Geometry check sheet. Reference: the model listing, model coordinates, mm. Give positions to 0.01 mm unless a question says otherwise; leave off trailing zeros. Write each loop counter-clockwise with the first axis right and the second up, starting at its lowest first coordinate (ties: lowest second). Pieces come first, ordered by that corner, then holes. Notation, with made-up numbers: (-24.5, 15.25) -> (-9.5, 15.25) arc R24 ccw to (-9.5, 30.25) -> close; hole circle Ø9 at (35.25, 30.25). An arc over 180 degrees is marked (long way). Write item = value, one per line. Start each with the question number.
1. Depth check by flat-ended pin: P1, Ø1.5, axis at x = -45.5, z = 27, coming from the +Y side. Enter the tip coordinate at first touch or a pass-through.
2. Thickness scan on line 1 along Z through (x, y) = (-50, -1.1); line 2 along Z through (x, y) = (-51, -0.8); line 3 along X through (y, z) = (-0.9, 45). Record the ranges inside material, lowest first.
3. Cross-section at A-A, the plane y = -0.65. Record the cut outline in (x, z) (3 decimals).
```python
from build123d import *

# Parameters (mm, degrees)
F0_W           = 95.9
F0_H           = 69.7
F1_DEPTH       = 1.54
F2_R           = 7
F3_D           = 2.8448
F3_CSINK_D     = 6.35
F3_CSINK_ANGLE = 90


with BuildPart() as f1:
    # F0 (on Front) → F1 (new body)
    with BuildSketch(Plane.XZ):
        with Locations((-8.388126269, 18.5557605668)):
            Rectangle(F0_W, F0_H)
    extrude(amount=F1_DEPTH)

    # F2
    f2_edges = [f1.edges().sort_by_distance(p)[0] for p in [
        (-56.338126, -0.77, -16.294239),
        (39.561874, -0.77, -16.294239),
        (39.561874, -0.77, 53.405761),
        (-56.338126, -0.77, 53.405761),
    ]]
    fillet(f2_edges, radius=F2_R)

    # F3 (through all)
    with Locations(Plane(origin=(0, 0, 0), x_dir=(1, 0, 0), z_dir=(0, 1, 0))):
        with Locations((-49.338126269, -46.4057605668), (32.561873731, -46.4057605668), (32.561873731, 9.2942394332), (-49.338126269, 9.2942394332)):
            CounterSinkHole(F3_D / 2, F3_CSINK_D / 2, counter_sink_angle=F3_CSINK_ANGLE)


solid = f1.part
```
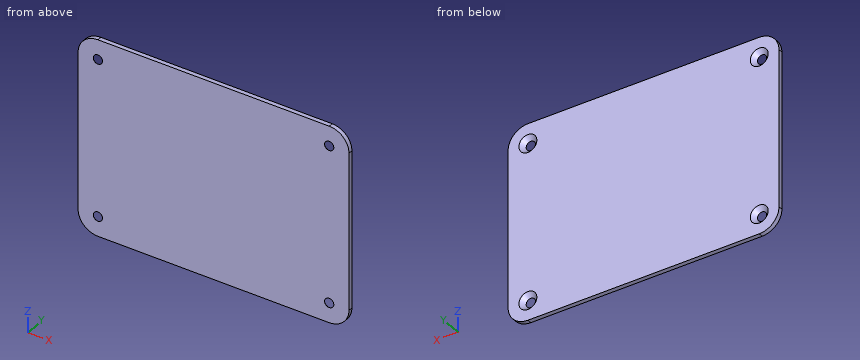
Answers:
q1.P1 = 0
q2.line_1 = -16.26 to -11.26, -7.33 to 44.44, 48.37 to 53.37
q2.line_2 = -16.09 to -10.99, -7.6 to 44.71, 48.1 to 53.21
q2.line_3 = -56.34 to -51.13, -47.55 to 30.77, 34.35 to 39.56
q3.outline = (-56.338, -9.294) arc R7 ccw to (-49.338, -16.294) -> (32.562, -16.294) arc R7 ccw to (39.562, -9.294) -> (39.562, 46.406) arc R7 ccw to (32.562, 53.406) -> (-49.338, 53.406) arc R7 ccw to (-56.338, 46.406) -> close; hole circle Ø5.05 at (-49.338, -9.294); hole circle Ø5.05 at (-49.338, 46.406); hole circle Ø5.05 at (32.562, -9.294); hole circle Ø5.05 at (32.562, 46.406)
